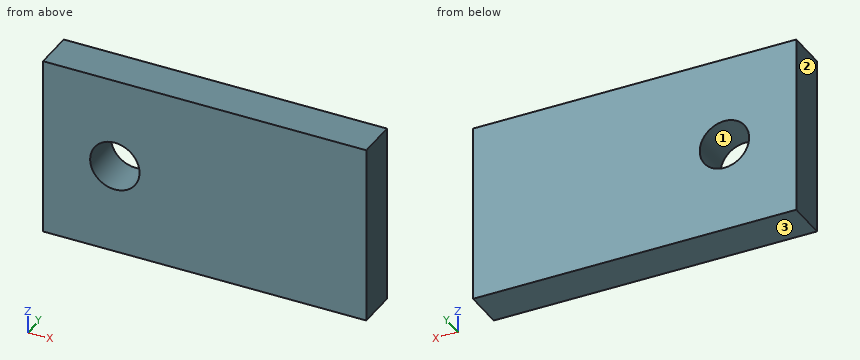
Autodesk Inventor part; units mm, degrees
ref_plane "YZ Plane" through (0, 0, 0) normal (1, 0, 0) x (0, 1, 0)
ref_plane "XZ Plane" through (0, 0, 0) normal (0, 1, 0) x (-1, 0, 0)
ref_plane "XY Plane" through (0, 0, 0) normal (0, 0, 1) x (1, 0, 0)
sketch "Sketch1" plane through (0, 0, 0) normal (0, 1, 0) x (-1, 0, 0)
  line L0 (0, 0) -> (36, 0)
  line L1 (36, 0) -> (36, -20)
  line L2 (36, -20) -> (0, -20)
  line L3 (0, -20) -> (0, 0)
  line L4 (36, -20) -> (28, -20)
  line L5 (0, -20) -> (8, -20)
  line L6 (28, -20) -> (28, 0)
  circle A0 centre (28, -10) radius 2.75
  dimension "d0" = 36
  dimension "d1" = 20
  dimension "d2" = 8
  dimension "d3" = 8
  dimension "d4" = 5.5
extrude "Extrusion1" add sketch "Sketch1" along normal blind 4.5 contours L0 L6 A0 L2 L3 | L0 L1 L2 L6 A0
properties part number "cable_retainer"
The listing builds one solid part. Answer for the finished solid, in the listing's coordinates (mm). Face numbers are marked on the shaded views. Give positions to 0.01 mm unless a question says otherwise; leave off trailing zeros. Order: outer loops, then holes, each group sorted by start corner. A loop starts at its lowest first (then second) coordinate and runs counter-clockwise, first axis right, second up. Notation, with made-up numbers: M 62,50.25 L 107,50.25 A5 cw 107,54.25 Z; hole C -5,78.25 d9. An arc over 180 degrees is marked long. Put each result on its own line as item: value. Start each with the question number.
Item 1: The part is cut by section A-A, the plane z = -10. Determine the outline of the cut face in (x, y).
Item 2: For a pull along Z with two mould halves and no side action, classify the marked faces 1, 2 and 3 as +Z half, -Z half, draft (parallel to the pull), parting line (faces both ways), or undercut.
Item 3: The part is cut by section B-B, the plane x = -28. Determine the outline of the cut face in (y, z).
Item 4: Find the intervals of material crossed by line 1 along X through (y, z) = (3.55, -10); line 2 along Z through (x, y) = (-28, 3.5); line 3 along X through (y, z) = (1.1, -11), in increasing order.
Item 5: The part is cut by section C-C, the plane y = 2.2. Determine the outline of the cut face in (x, z).
Answer key:
1. outline: M -36,0 L -30.75,0 L -30.75,4.5 L -36,4.5 Z; M -25.25,0 L 0,0 L 0,4.5 L -25.25,4.5 Z
2. face 1: undercut
2. face 2: draft
2. face 3: -Z half
3. outline: M 0,-20 L 4.5,-20 L 4.5,-12.75 L 0,-12.75 Z; M 0,-7.25 L 4.5,-7.25 L 4.5,0 L 0,0 Z
4. line 1: x = -36 to -30.75, -25.25 to 0
4. line 2: z = -20 to -12.75, -7.25 to 0
4. line 3: x = -36 to -30.56, -25.44 to 0
5. outline: M -36,-20 L 0,-20 L 0,0 L -36,0 Z; hole C -28,-10 d5.5
